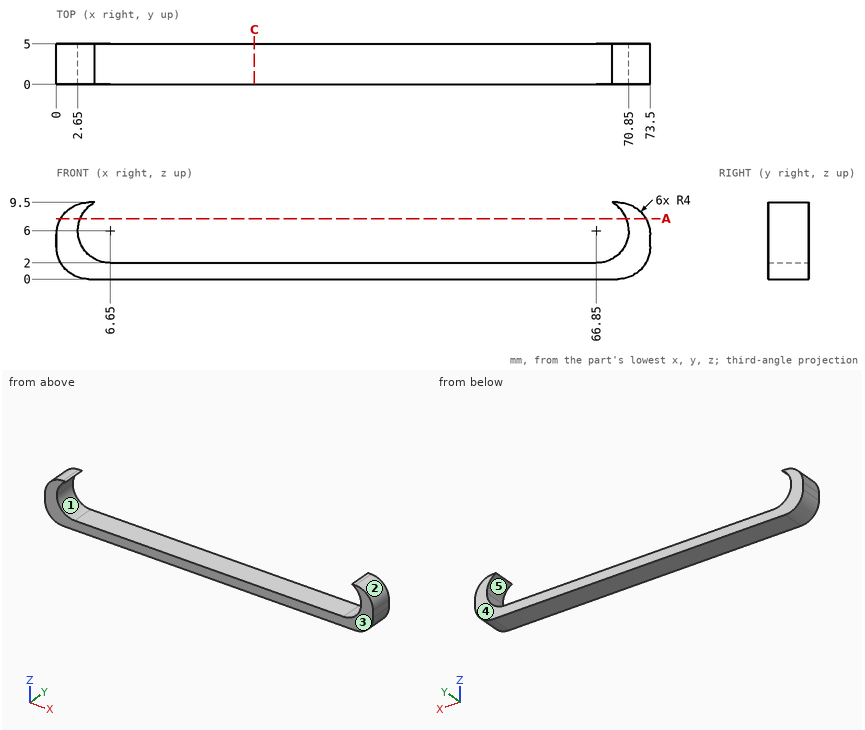
Can you work these out from the drawing? Everything is in mm from the part's minimum corner. A direction names the side the tool comes from. Coordinates: 2 decimals unless noted, no trailing zeros. Loops run counter-clockwise (first coordinate to the right, second up) from the corner with the lowest first, then second, coordinate; pieces in that order, holes last.
1. For P1, Ø1, axis at x = 14, z = 2, coming from the -Y side; P2, Ø3, axis at x = 12.5, y = 3, coming from the +Z side, each with a flat end and sliding along its axis, tell me the tip position at first contact or that it passes through.
2. I need wall thicknesses on L1, parallel to X at y = 4.4, z = 5.75; L2, parallel to Z at x = 40.5, y = 2.95; L3, parallel to X at y = 4.4, z = 2.5. Which ranges of each line are inside material? Lowest first, please.
3. Imagine slicing it at C-C, the plane x = 24.5. Please give me the cut outline in (y, z).
4. If we mould it in two halves opening along Z, with no side actions, what happens to the marked faces 1, 2 and 3? For each: pulls with the +Z half, pulls with the -Z half, needs draft (parallel to the pull), parting line crosses it, or undercut.
5. Imagine slicing it at A-A, the plane z = 7.5. Please give me the cut outline in (x, y).
6. For the marked faces 4 and 5, which set-ups out of +Z, -Z, +X, -X, +Y, -Y let a thin tool reach every point of the face, with its end or its side?
Taken from the geometry:
1. P1: stops at y = 0
1. P2: stops at z = 2
2. L1: x = 0.01 to 2.66, 70.84 to 73.49
2. L2: z = 0 to 2
2. L3: x = 0.29 to 4.71, 68.79 to 73.21
3. outline: (0, 0) - (5, 0) - (5, 2) - (0, 2) - close
4. face 1: undercut
4. face 2: pulls with the +Z half
4. face 3: needs draft
5. outline: (0.54, 0) - (2.94, 0) - (2.94, 5) - (0.54, 5) - close; (70.56, 0) - (72.96, 0) - (72.96, 5) - (70.56, 5) - close
6. face 4: +Z, -Z, +X, -X, +Y
6. face 5: +Y, -Y
